Model file for the job. Use its own axes, mm. Face numbers are marked on the shaded views. A direction names the side the tool comes from. Round coordinates to 2 decimals unless told otherwise and drop trailing zeros. Order: outer loops, then holes, each group sorted by start corner. A loop starts at its lowest first (then second) coordinate and runs counter-clockwise, first axis right, second up. Notation, with made-up numbers: (49.25, 52.25) - (89.25, 52.25) arc R17 ccw to (89.25, 77.25) - close; hole circle Ø9 at (52.5, 78.5). An arc over 180 degrees is marked (long way). Put each result on its own line as item: value. Start each with the question number.
Item 1: Probe probe 1 along X at (y, z) = (16.5, -10); probe 2 along Z at (x, y) = (0, 21.25); probe 3 along Z at (x, y) = (5, 38). List the from-to ranges inside material, lowest first.
Item 2: Which spindle directions (+Z, -Z, +X, -X, +Y, -Y) get a long thin tool onto all of the face, cutting with end or side? Do the marked faces 1 and 2. Say none if no direction does.
Item 3: Saw through at B-B on x = -15. List the corners of the cut face in (y, z).
Item 4: Saw through at D-D on x = -8. List the corners of the cut face in (y, z).
Item 5: Pin check, flat tips, straight feed: pin 1 Ø16 at (x, z) = (-11.5, -9) entering from +Y; pin 2 Ø6 at (x, y) = (9.5, 15.5) entering from -Z; pin 3 Ø18.5 at (x, y) = (-5.5, 30.5) entering from +Z. Stop position of each tip, or through.
Item 6: Saw through at C-C on z = -10. List the corners of the cut face in (x, y), plus the area to 3 significant figures.
Item 7: Saw through at A-A on y = 33. List the corners of the cut face in (x, z), plus the area to 3 significant figures.
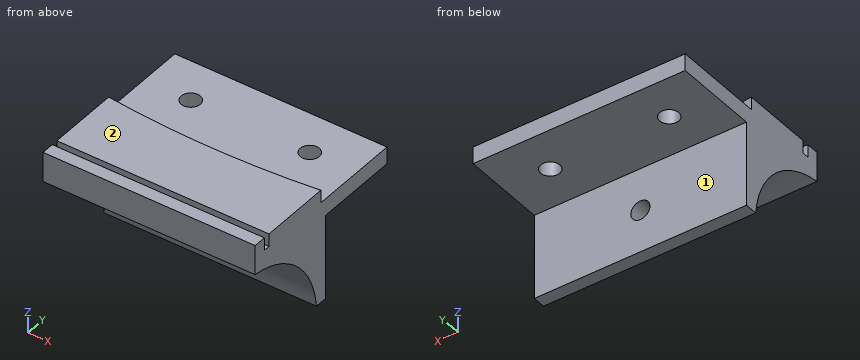
```python
from build123d import *

# Parameters (mm, degrees)
F0_R          = 2.25
F0_W          = 50
F0_H          = 1.5
F0_H_2        = 3
F1_DEPTH      = 4
F2_DEPTH      = 7
F4_DEPTH      = 25
F4_DEPTH_BACK = 25
F6_R          = 2.25
F7_DEPTH      = 23
F6_R_2        = 3.75
F8_DEPTH      = 10


with BuildPart() as f1:
    # F0 (on Top) → F1 (new body)
    with BuildSketch(Plane.XY):
        with BuildLine():
            Line((-25, 43), (-25, 21.42507))
            ThreePointArc((-25, 21.42507), (0, 20), (25, 21.42507))
            Line((25, 21.42507), (25, 43))
            Line((25, 43), (-25, 43))
        make_face()
        with Locations((-14.01787, 33)):
            Circle(F0_R, mode=Mode.SUBTRACT)
        with Locations((14.01787, 33)):
            Circle(F0_R, mode=Mode.SUBTRACT)
        with BuildLine():
            ThreePointArc((25, 21.42507), (0, 20), (-25, 21.42507))
            Line((-25, 21.42507), (-25, 4.5))
            Line((-25, 4.5), (25, 4.5))
            Line((25, 4.5), (25, 21.42507))
        make_face()
        with Locations((0, 3.75)):
            Rectangle(F0_W, F0_H)
        with Locations((0, 1.5)):
            Rectangle(F0_W, F0_H_2)
    extrude(amount=F1_DEPTH)

    # F0 (on Top) → F2 (join)
    with BuildSketch(Plane.XY):
        with BuildLine():
            ThreePointArc((25, 21.42507), (0, 20), (-25, 21.42507))
            Line((-25, 21.42507), (-25, 4.5))
            Line((-25, 4.5), (25, 4.5))
            Line((25, 4.5), (25, 21.42507))
        make_face()
        with Locations((0, 1.5)):
            Rectangle(F0_W, F0_H_2)
    extrude(amount=F2_DEPTH)

    # F3 (on Right) → F4 (join, two sides)
    with BuildSketch(Plane.YZ) as f4_sk:
        with BuildLine():
            Line((23, 0), (0, 0))
            ThreePointArc((0, 0), (13.557431, -6.442569), (20, -20))
            Line((20, -20), (23, -20))
            Line((23, -20), (23, 0))
        make_face()
    extrude(amount=F4_DEPTH)
    extrude(f4_sk.sketch, amount=-F4_DEPTH_BACK)

    # F6 (on Front) → F7 (cut, through all)
    with BuildSketch(Plane.XZ):
        with Locations((0, -10)):
            Circle(F6_R)
    extrude(amount=-F7_DEPTH, mode=Mode.SUBTRACT)

    # F6 (on Front) → F8 (cut)
    with BuildSketch(Plane.XZ):
        with Locations((0, -10)):
            Circle(F6_R_2)
        with Locations((0, -10)):
            Circle(F6_R, mode=Mode.SUBTRACT)
    extrude(amount=-F8_DEPTH, mode=Mode.SUBTRACT)


solid = f1.part
```
Results found:
1. probe 1: x = -25 to -2.25, 2.25 to 25
1. probe 2: z = -20 to -12.25, -7.75 to 4
1. probe 3: z = 0 to 4
2. face 1: -Z, +X, -X, +Y
2. face 2: +Z, +X, -X, +Y, -Y
3. outline: (0, 0) arc R22.39 cw to (20, -20) - (23, -20) - (23, 0) - (30.98, 0) - (30.98, 4) - (20.51, 4) - (20.51, 7) - (4.5, 7) - (4.5, 4) - (3, 4) - (3, 7) - (0, 7) - close; (35.02, 0) - (43, 0) - (43, 4) - (35.02, 4) - close
4. outline: (0, 0) arc R22.39 cw to (20, -20) - (23, -20) - (23, 0) - (43, 0) - (43, 4) - (20.15, 4) - (20.15, 7) - (4.5, 7) - (4.5, 4) - (3, 4) - (3, 7) - (0, 7) - close
5. pin 1: stops at y = 23
5. pin 2: stops at z = -13.92
5. pin 3: stops at z = 4
6. outline: (-25, 16.45) - (-2.25, 16.45) - (-2.25, 23) - (-25, 23) - close; (2.25, 16.45) - (25, 16.45) - (25, 23) - (2.25, 23) - close
6. area: 298 mm²
7. outline: (-25, 0) - (-16.27, 0) - (-16.27, 4) - (-25, 4) - close; (-11.77, 0) - (11.77, 0) - (11.77, 4) - (-11.77, 4) - close; (16.27, 0) - (25, 0) - (25, 4) - (16.27, 4) - close
7. area: 164 mm²
